from build123d import *

# Parameters (mm, degrees)
SKETCH1_W           = 40
SKETCH1_H           = 160
SKETCH1_R           = 10
BOSS_EXTRUDE1_DEPTH = 12
CUT_EXTRUDE3_REACH  = 85.331
SKETCH4_R           = 4
CUT_EXTRUDE4_REACH  = 163.691
SKETCH5_R           = 3
SKETCH6_R           = 10.25
CUT_EXTRUDE5_DEPTH  = 8


with BuildPart() as part:
    # Sketch1 → Boss-Extrude1 (new body)
    with BuildSketch(Plane(origin=(0, 0, 0), x_dir=(1, 0, 0), z_dir=(0, 1, 0))):
        Rectangle(SKETCH1_W, SKETCH1_H)
        with Locations(Location((0, 0, 0), (0, 0, 270))):
            Circle(SKETCH1_R, mode=Mode.SUBTRACT)
    extrude(amount=BOSS_EXTRUDE1_DEPTH)

    # Sketch4 → Cut-Extrude3 (cut, up to next)
    with BuildSketch(Plane(origin=(0, 12, 0), x_dir=(1, 0, 0), z_dir=(0, 1, 0)), mode=Mode.PRIVATE) as cut_extrude3_sk1:
        with Locations(Location((-10, 70, 0), (0, 0, 270))):
            Circle(SKETCH4_R)
    cut_extrude3_tool1 = extrude(cut_extrude3_sk1.sketch, amount=-CUT_EXTRUDE3_REACH, mode=Mode.PRIVATE) & part.part
    # Sketch4 → Cut-Extrude3 (cut, up to next)
    with BuildSketch(Plane(origin=(0, 12, 0), x_dir=(1, 0, 0), z_dir=(0, 1, 0)), mode=Mode.PRIVATE) as cut_extrude3_sk2:
        with Locations(Location((10, 70, 0), (0, 0, 270))):
            Circle(SKETCH4_R)
    cut_extrude3_tool2 = extrude(cut_extrude3_sk2.sketch, amount=-CUT_EXTRUDE3_REACH, mode=Mode.PRIVATE) & part.part
    cut_extrude3_1 = cut_extrude3_tool1.solids().sort_by_distance((-10, 12, -70))[0]
    add(cut_extrude3_1, mode=Mode.SUBTRACT)
    cut_extrude3_2 = cut_extrude3_tool2.solids().sort_by_distance((10, 12, -70))[0]
    add(cut_extrude3_2, mode=Mode.SUBTRACT)
    cut_extrude3 = cut_extrude3_1 + cut_extrude3_2  # Cut-Extrude3 as one shape, for the pattern or mirror that repeats it

    # Sketch5 → Cut-Extrude4 (cut, up to next)
    with BuildSketch(Plane(origin=(0, 0, -80), x_dir=(-1, 0, 0), z_dir=(0, 0, -1)), mode=Mode.PRIVATE) as cut_extrude4_sk1:
        with Locations((10, 6)):
            Circle(SKETCH5_R)
    cut_extrude4_tool1 = extrude(cut_extrude4_sk1.sketch, amount=-CUT_EXTRUDE4_REACH, mode=Mode.PRIVATE) & part.part
    # Sketch5 → Cut-Extrude4 (cut, up to next)
    with BuildSketch(Plane(origin=(0, 0, -80), x_dir=(-1, 0, 0), z_dir=(0, 0, -1)), mode=Mode.PRIVATE) as cut_extrude4_sk2:
        with Locations((-10, 6)):
            Circle(SKETCH5_R)
    cut_extrude4_tool2 = extrude(cut_extrude4_sk2.sketch, amount=-CUT_EXTRUDE4_REACH, mode=Mode.PRIVATE) & part.part
    cut_extrude4_1 = cut_extrude4_tool1.solids().sort_by_distance((-10, 6, -80))[0]
    add(cut_extrude4_1, mode=Mode.SUBTRACT)
    cut_extrude4_2 = cut_extrude4_tool2.solids().sort_by_distance((10, 6, -80))[0]
    add(cut_extrude4_2, mode=Mode.SUBTRACT)
    cut_extrude4 = cut_extrude4_1 + cut_extrude4_2  # Cut-Extrude4 as one shape, for the pattern or mirror that repeats it

    # Mirror1: Cut-Extrude3, Cut-Extrude4 across plane
    add(cut_extrude3.mirror(Plane.XY), mode=Mode.SUBTRACT)
    add(cut_extrude4.mirror(Plane.XY), mode=Mode.SUBTRACT)

    # Sketch6 → Cut-Extrude5 (cut)
    with BuildSketch(Plane(origin=(0, 12, 0), x_dir=(1, 0, 0), z_dir=(0, 1, 0))):
        with Locations(Location((0, 40, 0), (0, 0, 270))):
            Circle(SKETCH6_R)
        with Locations(Location((0, -40, 0), (0, 0, 270))):
            Circle(SKETCH6_R)
    extrude(amount=-CUT_EXTRUDE5_DEPTH, mode=Mode.SUBTRACT)


solid = part.part
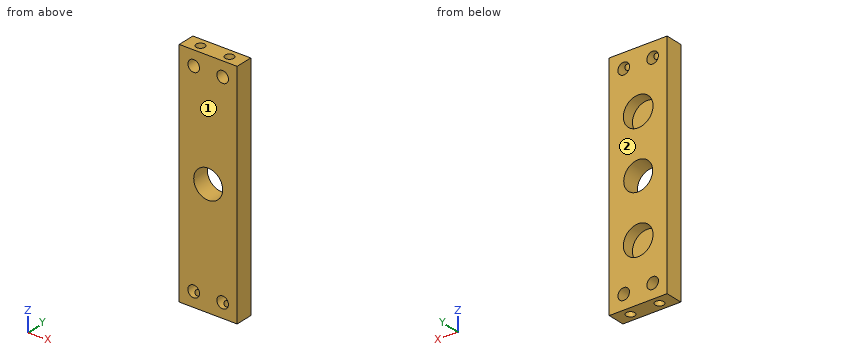
CAD build for the part. Positions are in the model's coordinates, mm. Face numbers are marked on the shaded views. Coordinates: 2 decimals unless noted, no trailing zeros. Order: outer loops, then holes, each group sorted by start corner. A loop starts at its lowest first (then second) coordinate and runs counter-clockwise, first axis right, second up. Notation, with made-up numbers: (76, 4) -> (132, 4) arc R7 cw to (132, 17) -> close; hole circle Ø7 at (-23.75, 16). An arc over 180 degrees is marked (long way). Answer in a Markdown table with one row per item.
1) Band-saw the part on C-C (x = -3). List the corners of the cut face in (y, z).
Check values:
| item | result |
|---|---|
| outline | (0, -80) -> (12, -80) -> (12, -49.8) -> (4, -49.8) -> (4, -30.2) -> (12, -30.2) -> (12, -9.54) -> (0, -9.54) -> close; (0, 9.54) -> (12, 9.54) -> (12, 30.2) -> (4, 30.2) -> (4, 49.8) -> (12, 49.8) -> (12, 80) -> (0, 80) -> close |
2) Band-saw the part on B-B (y = 6). List the corners of the cut face in (x, z).
Check values:
| item | result |
|---|---|
| outline | (-20, -80) -> (-13, -80) -> (-13, -72.65) arc R4 cw (long way) to (-7, -72.65) -> (-7, -80) -> (7, -80) -> (7, -72.65) arc R4 cw (long way) to (13, -72.65) -> (13, -80) -> (20, -80) -> (20, 80) -> (13, 80) -> (13, 72.65) arc R4 cw (long way) to (7, 72.65) -> (7, 80) -> (-7, 80) -> (-7, 72.65) arc R4 cw (long way) to (-13, 72.65) -> (-13, 80) -> (-20, 80) -> close; hole circle Ø20.5 at (0, -40); hole circle Ø20.5 at (0, 40); hole circle Ø20 at (0, 0) |
3) Band-saw the part on D-D (z = -40). List the corners of the cut face in (x, y), and give its area (3 significant figures).
Check values:
| item | result |
|---|---|
| outline | (-20, 0) -> (20, 0) -> (20, 12) -> (10.25, 12) -> (10.25, 4) -> (-10.25, 4) -> (-10.25, 12) -> (-20, 12) -> close |
| area | 316 mm2 |
4) Drill centre lines: line 1 (X direction, y = 8, z = 70); line 2 (X direction, y = 10, z = 40); line 3 (X direction, y = 4.25, z = 0). Where is each one in solid material? Low to high.
Check values:
| item | result |
|---|---|
| line 1 | -20 to -14, -6 to 6, 14 to 20 |
| line 2 | -20 to -10.25, 10.25 to 20 |
| line 3 | -20 to -10, 10 to 20 |
5) Band-saw the part on A-A (z = 70). List the corners of the cut face in (x, y), and give its area (3 significant figures).
Check values:
| item | result |
|---|---|
| outline | (-20, 0) -> (-14, 0) -> (-14, 12) -> (-20, 12) -> close; (-6, 0) -> (6, 0) -> (6, 12) -> (-6, 12) -> close; (14, 0) -> (20, 0) -> (20, 12) -> (14, 12) -> close |
| area | 288 mm2 |
6) Mould opens along Y. For the marked faces 1 and 2 say: pulls with the +Y half, pulls with the -Y half, needs draft (parallel to the pull), parting line crosses it, or undercut.
Check values:
| item | result |
|---|---|
| face 1 | pulls with the -Y half |
| face 2 | pulls with the +Y half |
7) Flat gauge pins, fed straight in: P1, Ø5.5, axis at x = 10, y = 6, coming from the -Z side; P2, Ø3.5, axis at x = -10, y = 6, coming from the +Z side; P3, Ø6, axis at x = 1.5, z = 40.5, coming from the +Y side. Where does each tip first touch, or does it go through?
Check values:
| item | result |
|---|---|
| P1 | z = -67.1 |
| P2 | z = 66.4 |
| P3 | y = 4 |
